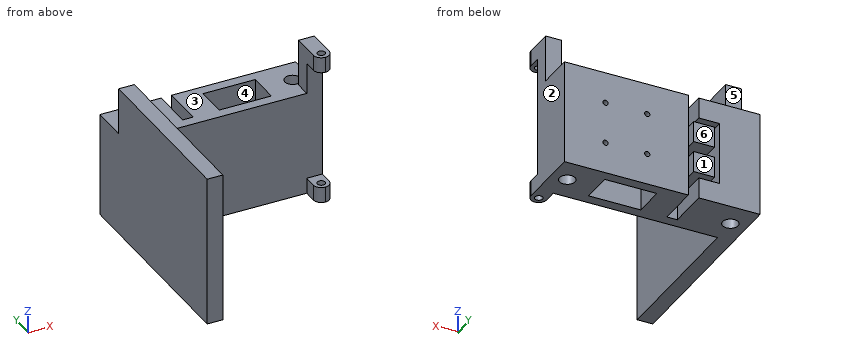
Autodesk Inventor part; units mm, degrees
ref_plane "YZ Plane" through (0, 0, 0) normal (1, 0, 0) x (0, 1, 0)
ref_plane "XZ Plane" through (0, 0, 0) normal (0, 1, 0) x (-1, 0, 0)
ref_plane "XY Plane" through (0, 0, 0) normal (0, 0, 1) x (1, 0, 0)
sketch "Sketch3" plane through (0, 0, 0) normal (0, 0, 1) x (1, 0, 0)
  line L0 (0, 0) -> (75, 0)
  line L1 (75, 0) -> (75, 20)
  line L2 (75, 20) -> (0, 20)
  line L3 (0, 20) -> (0, 0)
  circle A0 centre (6.25, 10) radius 3
  circle A1 centre (68.75, 10) radius 3
  line L4 (37.5, 16) -> (57.5, 16)
  line L5 (57.5, 16) -> (57.5, 4)
  line L6 (57.5, 4) -> (37.5, 4)
  line L7 (37.5, 4) -> (37.5, 16)
  dimension "d19" = 20
  dimension "d20" = 75
  dimension "d21" = 6
  dimension "d22" = 6
  dimension "d23" = 10
  dimension "d24" = 10
  dimension "d25" = 62.5
  dimension "d26" = 6.25
  dimension "d30" = 12
  dimension "d31" = 20
  dimension "d32" = 4
  dimension "d33" = 17.5
extrude "Extrusion3" add sketch "Sketch3" along normal blind 40
sketch "Sketch4" plane through (0, 20, 0) normal (0, 1, 0) x (1, 0, 0)
  line L0 (0, 0) -> (75, 0)
  line L1 (27.5, -40) -> (27.5, -20)
  line L2 (27.5, -20) -> (15.5, -20)
  line L3 (15.5, -20) -> (15.5, -32)
  line L4 (15.5, -32) -> (23.5, -32)
  line L5 (23.5, -32) -> (23.5, -40)
  line L6 (17.5, -22) -> (25.5, -22)
  line L7 (25.5, -22) -> (25.5, -30)
  line L8 (25.5, -30) -> (17.5, -30)
  line L9 (17.5, -30) -> (17.5, -22)
  line L10 (23.5, -40) -> (27.5, -40)
  line L11 (0, 0) -> (0, -40)
  line L12 (75, -40) -> (0, -40)
  line L13 (75, 0) -> (75, -40)
  line L14 (27.5, 0) -> (27.5, -20)
  line L15 (15.5, -20) -> (15.5, -8)
  line L16 (15.5, -8) -> (23.5, -8)
  line L17 (23.5, -8) -> (23.5, 0)
  line L18 (17.5, -18) -> (25.5, -18)
  line L19 (25.5, -18) -> (25.5, -10)
  line L20 (25.5, -10) -> (17.5, -10)
  line L21 (17.5, -10) -> (17.5, -18)
  line L22 (23.5, 0) -> (27.5, 0)
  dimension "d34" = 2
  dimension "d35" = 2
  dimension "d36" = 2
  dimension "d37" = 2
  dimension "d38" = 4
  dimension "d39" = 32
  dimension "d40" = 8
  dimension "d41" = 8
  dimension "d42" = 27.5
  dimension "d43" = 40
extrude "Extrusion4" cut sketch "Sketch4" against normal blind 16 contours L0 L14 L2 L15 L16 L17 | L5 L4 L3 L2 L1 L10
sketch "Sketch5" plane through (0, 0, 0) normal (0, -1, 0) x (1, 0, 0)
  line L0 (0, 0) -> (75, 0)
  line L1 (0, 40) -> (75, 40)
  line L2 (75, 0) -> (75, 40)
  line L3 (0, 0) -> (0, 40)
  line L4 (0, 40) -> (6, 40)
  line L5 (6, 40) -> (6, 58)
  line L6 (6, 58) -> (0, 58)
  line L7 (0, 58) -> (0, 40)
  line L8 (75, 40) -> (69, 40)
  line L9 (69, 40) -> (69, 58)
  line L10 (69, 58) -> (75, 58)
  line L11 (75, 58) -> (75, 40)
  dimension "d46" = 40
  dimension "d47" = 75
  dimension "d48" = 6
  dimension "d49" = 18
  dimension "d79" = 6
  dimension "d80" = 18
extrude "Extrusion5" add sketch "Sketch5" against normal blind 6 contours L7 L6 L5 L1 | L1 L9 L10 L11
sketch "Esquisse12" plane through (75, 20, 40) normal (0, 1, 0) x (1, 0, 0)
  circle A0 centre (-15.75, 12) radius 1
  line L0 (-47.5, 40) -> (-47.5, 0)
  line L1 (0, 0) -> (-47.5, 0)
  line L2 (0, 40) -> (0, 0)
  line L3 (0, 40) -> (-47.5, 40)
  circle A1 centre (-31.75, 12) radius 1
  circle A2 centre (-15.75, 28) radius 1
  circle A3 centre (-31.75, 28) radius 1
  line L4 (0, 6) -> (0, 52)
  line L5 (0, 0) -> (63, 0)
  line L6 (0, 40) -> (0, 0)
  point P0 (-75, 40)
  point P1 (-6, 0)
  point P2 (-75, 40)
  point P3 (69, 26.5)
  point P4 (0, 52)
  dimension "d122" = 2
  dimension "d123" = 16
  dimension "d124" = 16
  dimension "d125" = 15.75
  dimension "d126" = 47.5
  dimension "d127" = 40
  dimension "d128" = 12
  dimension "d129" = 47.5
extrude "Extrusion12" cut sketch "Esquisse12" against normal blind 5 contours A0 | A1 | A2 | A3
sketch "Esquisse13" plane through (0, 0, 0) normal (0, -1, 0) x (1, 0, 0)
  line L0 (0, 0) -> (0, 40)
  line L1 (0, 0) -> (6, 0)
  line L2 (6, 0) -> (6, 58)
  line L3 (6, 58) -> (0, 58)
  line L4 (0, 58) -> (0, 0)
extrude "Extrusion13" add sketch "Esquisse13" along normal blind 60
sketch "Esquisse14" plane through (6, 0, 0) normal (0, -1, 0) x (1, 0, 0)
  line L0 (63, 58) -> (63, 40)
  line L1 (69, 0) -> (69, 58)
  line L2 (63, 58) -> (69, 58)
  line L3 (69, 58) -> (69, 52)
  line L4 (69, 52) -> (63, 52)
  line L5 (63, 52) -> (63, 58)
  line L6 (0, 0) -> (69, 0)
  line L7 (69, 0) -> (63, 0)
  line L8 (63, 0) -> (63, 6)
  line L9 (63, 6) -> (69, 6)
  line L10 (69, 6) -> (69, 0)
  point P0 (-6, 0)
  dimension "d134" = 6
  dimension "d135" = 6
  dimension "d136" = 6
  dimension "d137" = 6
extrude "Extrusion14" add sketch "Esquisse14" along normal blind 8
sketch "Esquisse15" plane through (69, 6, 58) normal (0, 0, 1) x (1, 0, 0)
  circle A0 centre (3, -11) radius 1.5
  line L0 (6, -14) -> (0, -14)
  line L1 (-63, -6) -> (0, -6)
  line L2 (6, -6) -> (6, -14)
  point P0 (-69, -6)
  dimension "d140" = 3
  dimension "d141" = 3
  dimension "d142" = 6
  dimension "d143" = 8
  dimension "d144" = 3
extrude "Extrusion15" cut sketch "Esquisse15" against normal through all
fillet "Congé2" radius 3 4 edges at (69, -8, 55) (75, -8, 55) (75, -8, 3) (69, -8, 3)
equation "\"d22\" = d21"
equation "\"d23\" = 0.5 * d19"
equation "\"d24\" = 0.5 * d19"
equation "\"d26\" = 0.5 * d20 - 0.5 * d25"
equation "\"d32\" = 0.5 * d19 - 0.5 * d30"
equation "\"d33\" = 0.5 * d20 - d31"
equation "\"d35\" = d34"
equation "\"d36\" = d34"
equation "\"d37\" = d34"
equation "\"d38\" = 2 * d34"
equation "\"d40\" = 4 * d34"
equation "\"d41\" = 4 * d34"
equation "\"d79\" = d48"
equation "\"d80\" = d49"
equation "\"d125\" = 0.5 * d126 - 0.5 * d123"
equation "\"d128\" = 0.5 * d127 - 0.5 * d124"
equation "\"d135\" = d134"
equation "\"d136\" = d134"
equation "\"d137\" = d136"
equation "\"d144\" = 0.5 * d142"
properties part number "SupportPlateau" material "PC/ABS Plastic"
Read the model definition and answer for the solid it produces. Units are mm, in the model's axes. Face numbers are marked on the shaded views. A direction names the side the tool comes from. Give positions to 0.01 mm unless a question says otherwise; leave off trailing zeros. Loops run counter-clockwise (first coordinate to the right, second up) from the corner with the lowest first, then second, coordinate; pieces in that order, holes last. Notation, with made-up numbers: (26.25, 89.25) - (40.25, 89.25) arc R26 ccw to (40.25, 104.25) - close; hole circle Ø3 at (41.25, 2.25). An arc over 180 degrees is marked (long way). Answer as CSV lines item,"result". Start each with the question number.
1) Find section C-C (z = 43). Write down the section's boundary in (x, y), then the cut area to 3 significant figures.
2) Each of these flat-tipped pins is pushed along its axis until it touches: pin 1 Ø1.8 at (x, z) = (1.5, 53) entering from +Y; pin 2 Ø1.5 at (x, z) = (24.5, 33) entering from +Y; pin 3 Ø5 at (x, y) = (6.25, 10) entering from -Z; pin 4 Ø9 at (x, y) = (23, 11) entering from +Z. Where does it stop, or does it pass through?
3) Determine the mould class of the marked faces 1, 2 and 3 for opening direction X: released by +X, released by -X, zero draft, split by the parting line, or undercut.
4) Find section B-B (x = 51.5). Write down the section's boundary in (y, z), then the cut area to 3 significant figures.
5) Find section D-D (x = 43.25). Write down the section's boundary in (y, z), then the cut area to 3 significant figures.
6) Straight lines are drawn through the part: L1, parallel to Y at x = 45.5, z = 3.5; L2, parallel to X at y = 17.7, z = 12; L3, parallel to X at y = -27, z = 6.5. For each, find the intervals that lie inside material, in ascending order. Write a range as from..to.
7) Which of the six approach directions +Z, -Z, +X, -X, +Y, -Y give full straight-line access (tool end or side, diameter ignored) to the marked faces 4, 5 and 6?
8) Find section A-A (y = -1). Write down the section's boundary in (x, z).
Findings below:
1,outline,"(0, -60) - (6, -60) - (6, 6) - (0, 6) - close; (69, 0) - (75, 0) - (75, 6) - (69, 6) - close"
1,area,"432 mm^2"
2,pin 1,"y = 6"
2,pin 2,"y = 4"
2,pin 3,"through"
2,pin 4,"z = 40"
3,face 1,"zero draft"
3,face 2,"released by +X"
3,face 3,"undercut"
4,outline,"(0, 0) - (4, 0) - (4, 40) - (0, 40) - close; (16, 0) - (20, 0) - (20, 40) - (16, 40) - close"
4,area,"320 mm^2"
5,outline,"(0, 0) - (4, 0) - (4, 40) - (0, 40) - close; (16, 0) - (20, 0) - (20, 11) - (16, 11) - close; (16, 13) - (20, 13) - (20, 27) - (16, 27) - close; (16, 29) - (20, 29) - (20, 40) - (16, 40) - close"
5,area,"304 mm^2"
6,L1,"0..4, 16..20"
6,L2,"0..15.5, 17.5..25.5, 27.5..42.25, 44.25..58.25, 60.25..75"
6,L3,"0..6"
7,face 4,"+Z, -Z"
7,face 5,"+Z, +X, -X, +Y"
7,face 6,"+Z, -Z, +X, -X, +Y"
8,outline,"(0, 0) - (6, 0) - (6, 58) - (0, 58) - close; (69, 0) - (75, 0) - (75, 6) - (69, 6) - close; (69, 52) - (75, 52) - (75, 58) - (69, 58) - close"
